Read the model definition and answer for the solid it produces. Units are mm, in the model's axes. A direction names the side the tool comes from. Give positions to 0.01 mm unless a question says otherwise; leave off trailing zeros. Loops run counter-clockwise (first coordinate to the right, second up) from the corner with the lowest first, then second, coordinate; pieces in that order, holes last. Notation, with made-up numbers: (52.25, 2.5) - (57.25, 2.5) arc R29 cw to (57.25, 34.5) - close; hole circle Ø7 at (70, 69.5). An arc over 180 degrees is marked (long way). Write item = value, one per line.
```python
from build123d import *

# Parameters (mm, degrees)
F0_R     = 25.4
F0_R_2   = 12.7
F1_DEPTH = 76.2
F2_DEPTH = 76.2
F3_W     = 20.32
F3_H     = 38.1
F4_DEPTH = 177.8
F5_D     = 25.4
F5_DEPTH = 76.201
F6_D     = 25.4


with BuildPart() as f1:
    # F0 (on Front) → F1 (new body)
    with BuildSketch(Plane.XZ):
        Circle(F0_R)
        Circle(F0_R_2, mode=Mode.SUBTRACT)
    extrude(amount=F1_DEPTH)

    # F2 (add): a face of the model
    f2_faces = [f1.faces().sort_by_distance(p)[0] for p in [
        (-24.6815795103, 0, 0),
    ]]
    extrude(f2_faces, amount=F2_DEPTH)

    # F3 (on Right) → F4 (join)
    with BuildSketch(Plane.YZ):
        Rectangle(F3_W, F3_H)
    extrude(amount=F4_DEPTH)

    # F5 (through all, one way)
    with BuildSketch(Plane(origin=(0, 0, 0), x_dir=(1, 0, 0), z_dir=(0, 1, 0))):
        with Locations((0, 0)):
            Circle(F5_D / 2)
    extrude(amount=-F5_DEPTH, mode=Mode.SUBTRACT)

    # F6 (through all)
    with Locations(Plane.XZ):
        with Locations((0, 0)):
            Hole(F6_D / 2)


solid = f1.part
```
1) A tool of negligible diameter and unlimited length cuts with its end or side. For faces 1 (the face through (96, 0, 19.05)), 2 (the face through (5, 76.2, 12)), 3 (the face through (96, 0, -19.05)), from which of +Z, -Z, +X, -X, +Y, -Y can it reach the whole face along a straight path? Write none if from no direction.
Output:
face_1 = +Z, +X, +Y, -Y
face_2 = +Z, -Z, +X, -X, +Y
face_3 = -Z, +X, +Y, -Y
2) Each of these flat-tipped pins is pushed along its axis until it touches: P1, Ø1, axis at x = 119, y = 5, coming from the +Z side; P2, Ø11.5, axis at x = 109.5, z = 7, coming from the -Y side; P3, Ø6, axis at x = 129.5, y = 0.5, coming from the -Z side; P4, Ø2, axis at x = 28, y = 39, coming from the +Z side. Where does it stop, or does it pass through?
Output:
P1 = 19.05
P2 = -10.16
P3 = -19.05
P4 = through
3) Find the intervals of material crossed by probe 1 along Z at (x, y) = (108.5, -2); probe 2 along Y at (x, z) = (105.5, 11); probe 3 along X at (y, z) = (8, 9.5), in increasing order.
Output:
probe_1 = -19.05 to 19.05
probe_2 = -10.16 to 10.16
probe_3 = -23.56 to -8.43, 8.43 to 177.8
4) A cutting plane is placed at B-B on y = 54.5. Determine the outline of the cut face in (x, z).
Output:
outline = circle Ø50.8 at (0, 0); hole circle Ø25.4 at (0, 0)
5) A cutting plane is placed at D-D on x = 63. Determine the outline of the cut face in (y, z).
Output:
outline = (-10.16, -19.05) - (10.16, -19.05) - (10.16, 19.05) - (-10.16, 19.05) - close
6) A cutting plane is placed at C-C on x = 21.5. Determine the outline of the cut face in (y, z).
Output:
outline = (-76.2, -13.52) - (-10.16, -13.52) - (-10.16, -19.05) - (10.16, -19.05) - (10.16, -13.52) - (76.2, -13.52) - (76.2, 13.52) - (10.16, 13.52) - (10.16, 19.05) - (-10.16, 19.05) - (-10.16, 13.52) - (-76.2, 13.52) - close
7) A cutting plane is placed at A-A on z = -8. Determine the outline of the cut face in (x, y), then the cut area to 3 significant figures.
Output:
outline = (-24.11, -76.2) - (-9.86, -76.2) - (-9.86, 76.2) - (-24.11, 76.2) - close; (9.86, -76.2) - (24.11, -76.2) - (24.11, -10.16) - (177.8, -10.16) - (177.8, 10.16) - (24.11, 10.16) - (24.11, 76.2) - (9.86, 76.2) - close
area = 7,460 mm²
